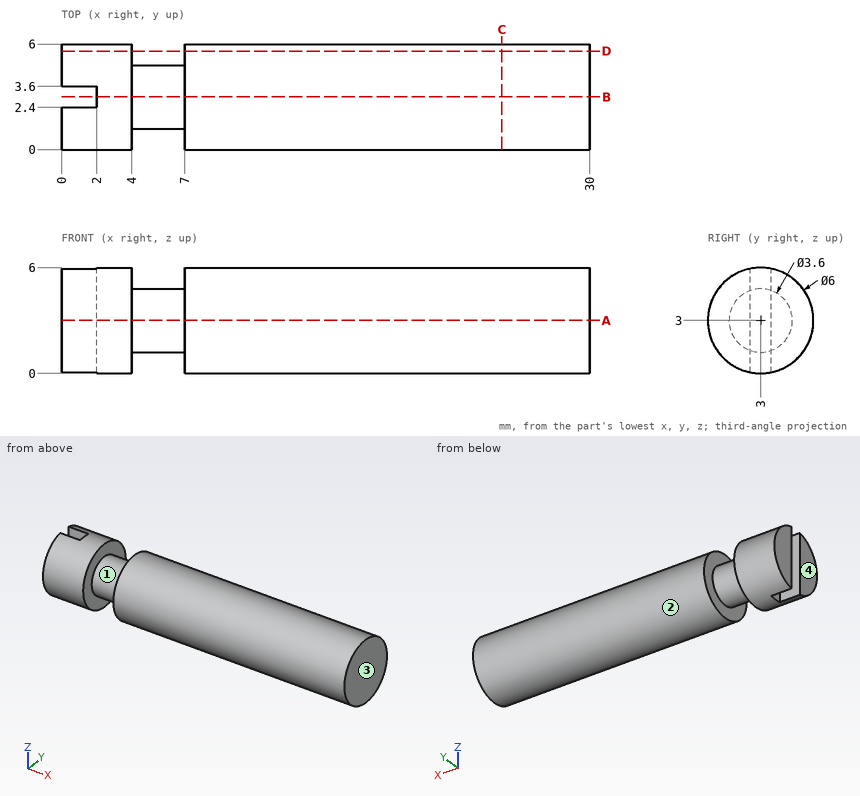
Design review of the part shown in the three views and the two pictorial views. Dimensions are in mm from the part's minimum x, y and z. Round coordinates to 2 decimals unless told otherwise and drop trailing zeros. Write each loop counter-clockwise with the first axis right and the second up, starting at its lowest first coordinate (ties: lowest second). Pieces come first, ordered by that corner, then holes. Notation, with made-up numbers: (-7, 73.25) -> (49, 73.25) arc R26 ccw to (49, 99.25) -> close; hole circle Ø8 at (-27.5, -7). An arc over 180 degrees is marked (long way). Answer as a JSON object with one key per item and string values.
1. We need section B-B on y = 3. State the section outline as (x, z) points.
Results found:
{"outline": "(2, 0) -> (4, 0) -> (4, 1.2) -> (7, 1.2) -> (7, 0) -> (30, 0) -> (30, 6) -> (7, 6) -> (7, 4.8) -> (4, 4.8) -> (4, 6) -> (2, 6) -> close"}
2. The part is to be moulded in two halves that separate along X. For the marked faces 1, 2, 3 and 4, say which applies: pulls with the +X half, pulls with the -X half, needs draft (parallel to the pull), parting line crosses it, or undercut.
Results found:
{"face 1": "undercut", "face 2": "needs draft", "face 3": "pulls with the +X half", "face 4": "pulls with the -X half"}
3. To check wall thickness, follow line 1 along X through (y, z) = (5.6, 4.15); line 2 along Z through (x, y) = (5.5, 2.9); line 3 along Y through (x, z) = (28.5, 3.2). State the ranges of each line that lie inside material, in increasing order.
Results found:
{"line 1": "x = 0 to 4, 7 to 30", "line 2": "z = 1.2 to 4.8", "line 3": "y = 0.01 to 5.99"}
4. We need section A-A on z = 3. State the section outline as (x, y) points.
Results found:
{"outline": "(0, 0) -> (4, 0) -> (4, 1.2) -> (7, 1.2) -> (7, 0) -> (30, 0) -> (30, 6) -> (7, 6) -> (7, 4.8) -> (4, 4.8) -> (4, 6) -> (0, 6) -> (0, 3.6) -> (2, 3.6) -> (2, 2.4) -> (0, 2.4) -> close"}
5. We need section D-D on y = 5.6. State the section outline as (x, z) points.
Results found:
{"outline": "(0, 1.5) -> (4, 1.5) -> (4, 4.5) -> (0, 4.5) -> close; (7, 1.5) -> (30, 1.5) -> (30, 4.5) -> (7, 4.5) -> close"}
6. Clearance check with flat-ended pins moving along their axes: pin 1 (0.6 mm diameter, centred on x = 1, z = 4, fed in from -Y); pin 2 (3 mm diameter, centred on x = 16.5, y = 1, fed in from +Z); pin 3 (0.6 mm diameter, centred on y = 3, z = 3, fed in from -X). State where each tip first meets the part, or that it passes through.
Results found:
{"pin 1": "stops at y = 0.08", "pin 2": "stops at z = 5.96", "pin 3": "stops at x = 2"}
7. We need section C-C on x = 25. State the section outline as (y, z) points.
Results found:
{"outline": "circle Ø6 at (3, 3)"}
